CAD build for the part. Positions are in the model's coordinates, mm. Face numbers are marked on the shaded views. A direction names the side the tool comes from. Give positions to 0.01 mm unless a question says otherwise; leave off trailing zeros. Loops run counter-clockwise (first coordinate to the right, second up) from the corner with the lowest first, then second, coordinate; pieces in that order, holes last.
```python
from build123d import *

# Parameters (mm, degrees)
SKETCH1_R           = 12.5
BOSS_EXTRUDE1_DEPTH = 7.5
SKETCH2_W           = 35
SKETCH2_H           = 8.580767914
BOSS_EXTRUDE2_DEPTH = 25
SKETCH3_W           = 25
SKETCH3_H           = 8.580767914
CUT_EXTRUDE1_DEPTH  = 20
SKETCH4_R           = 5
BOSS_EXTRUDE3_DEPTH = 3.75
SKETCH5_R           = 5
BOSS_EXTRUDE4_DEPTH = 3.75
CHAMFER1_SIZE       = 5
CHAMFER2_SIZE       = 5


with BuildPart() as part:
    # Sketch1 → Boss-Extrude1 (new body)
    with BuildSketch(Plane(origin=(0, 0, 0), x_dir=(1, 0, 0), z_dir=(0, 1, 0))):
        Circle(SKETCH1_R)
    extrude(amount=BOSS_EXTRUDE1_DEPTH)

    # Sketch2 → Boss-Extrude2 (add)
    with BuildSketch(Plane(origin=(0, 7.5, 0), x_dir=(1, 0, 0), z_dir=(0, 1, 0))):
        Rectangle(SKETCH2_W, SKETCH2_H)
    extrude(amount=BOSS_EXTRUDE2_DEPTH)

    # Sketch3 → Cut-Extrude1 (cut)
    with BuildSketch(Plane(origin=(0, 32.5, 0), x_dir=(1, 0, 0), z_dir=(0, 1, 0))):
        Rectangle(SKETCH3_W, SKETCH3_H)
    extrude(amount=-CUT_EXTRUDE1_DEPTH, mode=Mode.SUBTRACT)

    # Sketch4 → Boss-Extrude3 (add)
    with BuildSketch(Plane(origin=(-12.5, 0, 0), x_dir=(0, 0, -1), z_dir=(1, 0, 0))):
        with Locations((0, 27.5)):
            Circle(SKETCH4_R)
    extrude(amount=BOSS_EXTRUDE3_DEPTH)

    # Sketch5 → Boss-Extrude4 (add)
    with BuildSketch(Plane.ZY.offset(-12.5)):
        with Locations((0, 27.5)):
            Circle(SKETCH5_R)
    extrude(amount=BOSS_EXTRUDE4_DEPTH)

    # Chamfer1
    chamfer1_edges = [part.edges().sort_by_distance(p)[0] for p in [
        (-12.5, 12.5, 0),
    ]]
    chamfer(chamfer1_edges, length=CHAMFER1_SIZE)

    # Chamfer2
    chamfer2_edges = [part.edges().sort_by_distance(p)[0] for p in [
        (12.5, 12.5, 0),
    ]]
    chamfer(chamfer2_edges, length=CHAMFER2_SIZE)


solid = part.part
```
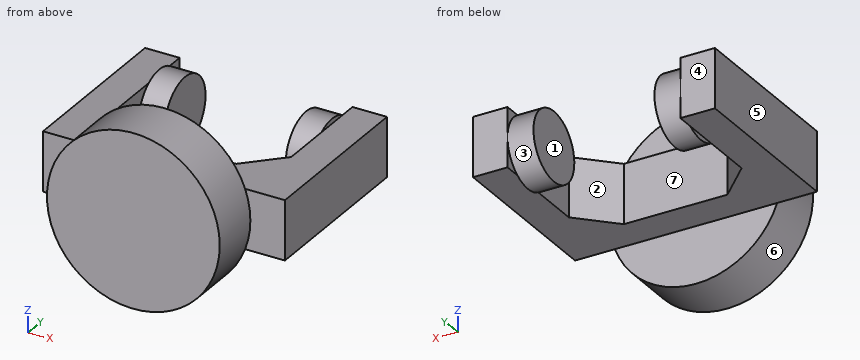
1. Saw through at C-C, the plane y = 15.5. List the corners of the cut face in (x, z).
Responses:
outline: (-17.5, -4.29) - (-10.5, -4.29) - (-10.5, 4.29) - (-17.5, 4.29) - close; (10.5, -4.29) - (17.5, -4.29) - (17.5, 4.29) - (10.5, 4.29) - close
2. Pull direction X, two halves, no side cores. Call the marked faces 4, 5, 6 and 7: released by +X, released by -X, zero draft, split by the parting line, or undercut.
Responses:
face 4: zero draft
face 5: released by -X
face 6: split by the parting line
face 7: undercut
3. Saw through at D-D, the plane x = 0. List the corners of the cut face in (y, z), and give its area (3 significant figures).
Responses:
outline: (0, -12.5) - (7.5, -12.5) - (7.5, -4.29) - (12.5, -4.29) - (12.5, 4.29) - (7.5, 4.29) - (7.5, 12.5) - (0, 12.5) - close
area: 230 mm2
4. Probe line 1 along X through (y, z) = (21.5, 3); line 2 along Z through (x, y) = (13.5, 19); line 3 along Y through (x, z) = (-3, -2.5). List the from-to ranges inside material, lowest first.
Responses:
line 1: x = -17.5 to -12.5, 12.5 to 17.5
line 2: z = -4.29 to 4.29
line 3: y = 0 to 12.5
5. Saw through at A-A, the plane y = 27.5. List the corners of the cut face in (x, z), and give its area (3 significant figures).
Responses:
outline: (-17.5, -4.29) - (-12.5, -4.29) - (-12.5, -5) - (-8.75, -5) - (-8.75, 5) - (-12.5, 5) - (-12.5, 4.29) - (-17.5, 4.29) - close; (8.75, -5) - (12.5, -5) - (12.5, -4.29) - (17.5, -4.29) - (17.5, 4.29) - (12.5, 4.29) - (12.5, 5) - (8.75, 5) - close
area: 161 mm2
6. Tool access for the marked faces 1, 2 and 3: list every direction of +Z, -Z, +X, -X, +Y, -Y with a clear straight run to the whole face (end or side of a thin tool).
Responses:
face 1: +Z, -Z, +Y
face 2: +Z, -Z
face 3: none
7. Drop flat-ended pins along their axis: pin 1 (1.7 mm diameter, centred on x = 14.5, z = -0.5, fed in from -Y); pin 2 (2 mm diameter, centred on x = -11.5, z = 6.5, fed in from +Y); pin 3 (4.5 mm diameter, centred on x = -1, z = -2, fed in from +Y). Give the stop position or say it passes through.
Responses:
pin 1: stops at y = 7.5
pin 2: stops at y = 7.5
pin 3: stops at y = 12.5
8. Saw through at B-B, the plane x = -10. List the corners of the cut face in (y, z).
Responses:
outline: (0, -7.5) - (7.5, -7.5) - (7.5, -4.29) - (15, -4.29) - (15, 4.29) - (7.5, 4.29) - (7.5, 7.5) - (0, 7.5) - close; circle Ø10 at (27.5, 0)
